```python
from build123d import *

# Parameters (mm, degrees)
BOSS_EXTRUDE1_DEPTH = 19.05
FILLET1_R           = 2.54
FILLET2_R           = 0.635


with BuildPart() as part:
    # Sketch1 → Boss-Extrude1 (new body)
    with BuildSketch(Plane.XY):
        Polygon((-25.398341139, -10.622644211), (0, -10.622644211), (0, 10.622644211), (-25.398341139, 10.332355789), (-25.398341139, 7.157355789), (-3.175, 7.411355789), (-3.175, 7.157355789), (-3.175, 2.077355789), (-25.398341139, 2.077355789), align=None)
    extrude(amount=BOSS_EXTRUDE1_DEPTH)

    # Fillet1
    fillet1_edges = [part.edges().sort_by_distance(p)[0] for p in [
        (-12.69917057, 10.4775, 0),
        (0, 0, 0),
        (-12.69917057, -10.622644211, 0),
        (-25.398341139, -4.272644211, 0),
        (-25.398341139, 10.332355789, 9.525),
        (0, 10.622644211, 9.525),
        (0, -10.622644211, 9.525),
        (-25.398341139, -10.622644211, 9.525),
        (-25.398341139, -4.272644211, 19.05),
        (-12.69917057, -10.622644211, 19.05),
        (0, 0, 19.05),
        (-12.69917057, 10.4775, 19.05),
        (-25.398341139, 8.744855789, 19.05),
        (-25.398341139, 8.744855789, 0),
    ]]
    fillet(fillet1_edges, radius=FILLET1_R)

    # Fillet2
    fillet2_edges = [part.edges().sort_by_distance(p)[0] for p in [
        (-13.01667057, 7.298871158, 0),
        (-25.398341139, 7.157355789, 9.525),
        (-24.654392364, 7.165858695, 18.306051224),
        (-24.654392364, 7.165858695, 0.743948776),
        (-13.01667057, 7.298871158, 19.05),
    ]]
    fillet(fillet2_edges, radius=FILLET2_R - 0.0004)  # a hair under: the kernel refuses the full size


solid = part.part
```
Model file for the job. Use its own axes, mm. A direction names the side the tool comes from. Coordinates: 2 decimals unless noted, no trailing zeros. Loops run counter-clockwise (first coordinate to the right, second up) from the corner with the lowest first, then second, coordinate; pieces in that order, holes last. Notation, with made-up numbers: (10, 60) - (24, 60) arc R24 cw to (24, 87) - close; hole circle Ø9 at (-18.5, 57). An arc over 180 degrees is marked (long way). Answer as a JSON object with one key per item and string values. Group by question number.
(1) Probe line 1 along X through (y, z) = (2.75, 3.5) (3 decimals); line 2 along Y through (x, z) = (-23.75, 7.75); line 3 along Y through (x, z) = (-20.25, 8.25). List the from-to ranges inside material, lowest first.
(2) Flat gauge pins, fed straight in: pin 1 (4 mm diameter, centred on x = -20, y = 5.5, fed in from +Z); pin 2 (2 mm diameter, centred on x = -21.5, z = 10.5, fed in from +Y); pin 3 (1 mm diameter, centred on y = 6.5, z = 17, fed in from -X) (3 decimals). Where does each tip first touch, or does it go through?
(3) Cut at A-A (z = 8.25). Give the cut face in (x, y) (3 decimals).
(4) Cut at B-B (y = 3). Give the cut face in (x, z) (3 decimals).
(5) Tool access for faces 1 (the face through (0, 0, 9)), 2 (the face through (-14, 2.077, 9)): list every direction of +Z, -Z, +X, -X, +Y, -Y with a clear straight run to the whole face (end or side of a thin tool).
(6) Two-plate mould, pull along Y, no slides. Class faces 3 (the face through (-13.15, 7.49, 18.87)), 4 (the face through (-12.86, 9.75, 18.29)), 5 (the face through (-0.724, 0.098, 18.286)): released by +Y, released by -Y, zero draft, split by the parting line, or undercut.
Geometry says:
{
 "1": {"line 1": "x = -3.175 to 0", "line 2": "y = -10.46 to 2.08, 7.18 to 10.2", "line 3": "y = -10.62 to 2.08, 7.22 to 10.39"},
 "2": {"pin 1": "stops at z = 18.94", "pin 2": "stops at y = 10.39", "pin 3": "stops at x = -3.175"},
 "3": {"outline": "(-25.398, -8.083) arc R2.54 ccw to (-22.858, -10.623) - (-2.54, -10.623) arc R2.54 ccw to (0, -8.083) - (0, 8.053) arc R2.54 ccw to (-2.569, 10.593) - (-22.887, 10.361) arc R2.54 ccw to (-25.398, 7.821) - (-25.398, 7.799) arc R0.635 ccw to (-24.756, 7.165) - (-3.175, 7.411) - (-3.175, 2.077) - (-25.398, 2.077) - close"},
 "4": {"outline": "(-3.175, 0) - (-2.54, 0) arc R2.54 ccw to (0, 2.54) - (0, 16.51) arc R2.54 ccw to (-2.54, 19.05) - (-3.175, 19.05) - close"},
 "5": {"face 1": "+Z, -Z, +X, +Y, -Y", "face 2": "+Z, -Z, -X"},
 "6": {"face 3": "undercut", "face 4": "released by +Y", "face 5": "zero draft"}
}
